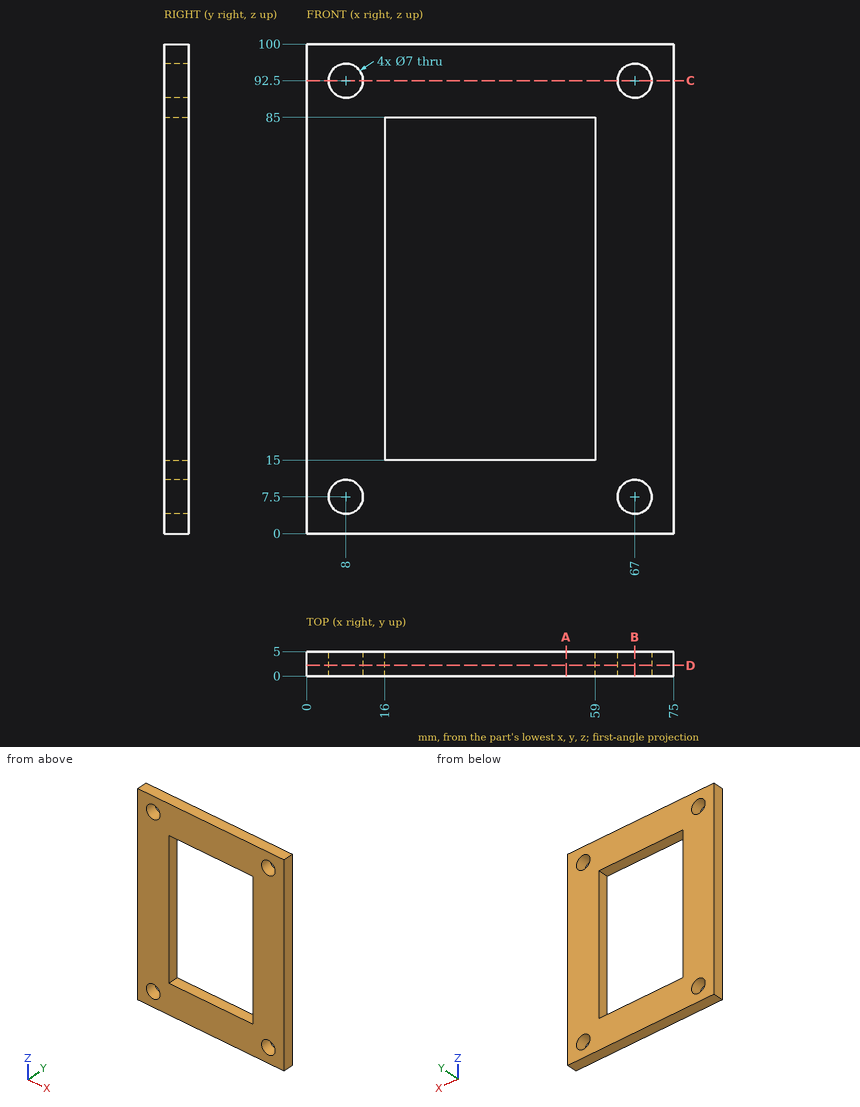
Design review of the part shown in the three views and the two pictorial views. Dimensions are in mm from the part's minimum x, y and z. Round coordinates to 2 decimals unless told otherwise and drop trailing zeros. Loops run counter-clockwise (first coordinate to the right, second up) from the corner with the lowest first, then second, coordinate; pieces in that order, holes last. Notation, with made-up numbers: (-35, 49.5) - (-16, 49.5) arc R5 ccw to (-16, 55.5) - close; hole circle Ø10 at (16, -23). An arc over 180 degrees is marked (long way). Answer as CSV lines item,"result".
(1) Consider section C-C on z = 92.5. Give the boundary of the cut face in (x, y), then the cut area to 3 significant figures.
Checked values:
outline,"(0, 0) - (4.5, 0) - (4.5, 5) - (0, 5) - close; (11.5, 0) - (63.5, 0) - (63.5, 5) - (11.5, 5) - close; (70.5, 0) - (75, 0) - (75, 5) - (70.5, 5) - close"
area,"305 mm2"
(2) Consider section B-B on x = 67. Give the boundary of the cut face in (y, z).
Checked values:
outline,"(0, 0) - (5, 0) - (5, 4) - (0, 4) - close; (0, 11) - (5, 11) - (5, 89) - (0, 89) - close; (0, 96) - (5, 96) - (5, 100) - (0, 100) - close"
(3) Wall thickness on line 1 (Z direction, x = 8, y = 4.05); line 2 (X direction, y = 2.45, z = 92.5); line 3 (Z direction, x = 54, y = 0.35): over which ranges is each line inside the solid? List them lowest first.
Checked values:
line 1,"z = 0 to 4, 11 to 89, 96 to 100"
line 2,"x = 0 to 4.5, 11.5 to 63.5, 70.5 to 75"
line 3,"z = 0 to 15, 85 to 100"
(4) Insertion check: P1, Ø2.5, axis at y = 3.5, z = 39, coming from the -X side. The pin has a flat end and moves straight along its axis. Give the tip position at first contact, or say it passes through.
Checked values:
P1,"stops at x = 0"
(5) Consider section D-D on y = 2.15. Give the boundary of the cut face in (x, z).
Checked values:
outline,"(0, 0) - (75, 0) - (75, 100) - (0, 100) - close; hole circle Ø7 at (8, 7.5); hole circle Ø7 at (8, 92.5); hole (16, 15) - (59, 15) - (59, 85) - (16, 85) - close; hole circle Ø7 at (67, 7.5); hole circle Ø7 at (67, 92.5)"
(6) Consider section A-A on x = 53. Give the boundary of the cut face in (y, z), then the cut area to 3 significant figures.
Checked values:
outline,"(0, 0) - (5, 0) - (5, 15) - (0, 15) - close; (0, 85) - (5, 85) - (5, 100) - (0, 100) - close"
area,"150 mm2"
